Can you work these out from the model? Positions are in its coordinate system, mm. A direction names the side the tool comes from. Give positions to 0.01 mm unless a question says otherwise; leave off trailing zeros. Loops run counter-clockwise (first coordinate to the right, second up) from the corner with the lowest first, then second, coordinate; pieces in that order, holes last. Notation, with made-up numbers: (-9, -26) - (33, -26) arc R15 cw to (33, -6) - close; hole circle Ø7 at (19.25, 39.5). An arc over 180 degrees is marked (long way). Answer in a Markdown table with one row per item.
from build123d import *

# Parameters (mm, degrees)
BOSS_EXTRUDE1_DEPTH = 1500
CUT_EXTRUDE1_DEPTH  = 100
SKETCH3_R           = 50
CUT_EXTRUDE2_DEPTH  = 50
SKETCH4_R           = 25
CUT_EXTRUDE3_DEPTH  = 25


with BuildPart() as part:
    # Sketch1 → Boss-Extrude1 (new body)
    with BuildSketch(Plane(origin=(0, 0, 0), x_dir=(0, 0, -1), z_dir=(1, 0, 0))):
        with BuildLine():
            Line((-50, 50), (-50, -50))
            ThreePointArc((-50, -50), (0, -100), (50, -50))
            Line((50, -50), (50, 50))
            ThreePointArc((50, 50), (0, 100), (-50, 50))
        make_face()
    extrude(amount=-BOSS_EXTRUDE1_DEPTH)

    # Sketch2 → Cut-Extrude1 (cut)
    with BuildSketch(Plane.XY.offset(50)):
        with BuildLine():
            Line((-100.5, 100), (0, 100))
            Line((0, 100), (0, -100))
            Line((0, -100), (-100.5, -100))
            ThreePointArc((-100.5, -100), (-0.5, 0), (-100.5, 100))
        make_face()
    extrude(amount=-CUT_EXTRUDE1_DEPTH, mode=Mode.SUBTRACT)

    # Sketch3 → Cut-Extrude2 (cut)
    with BuildSketch(Plane.XY.offset(50)):
        with Locations((-100, 0)):
            Circle(SKETCH3_R)
    extrude(amount=-CUT_EXTRUDE2_DEPTH, mode=Mode.SUBTRACT)

    # Sketch4 → Cut-Extrude3 (cut)
    with BuildSketch(Plane.ZY.offset(1500)):
        with Locations((0, 50)):
            Circle(SKETCH4_R)
        with Locations((0, -50)):
            Circle(SKETCH4_R)
    extrude(amount=-CUT_EXTRUDE3_DEPTH, mode=Mode.SUBTRACT)


solid = part.part
Q1. For pin 1 (10 mm diameter, centred on x = -464.5, z = -15.5, fed in from +Y); pin 2 (3 mm diameter, centred on y = -28, z = 0.5, fed in from -X); pin 3 (1 mm diameter, centred on y = -2, z = 13.5, fed in from +X), each with a flat end and sliding along its axis, tell me the tip position at first contact or that it passes through.
Checked values:
| item | result |
|---|---|
| pin 1 | stops at y = 98.89 |
| pin 2 | stops at x = -1475 |
| pin 3 | stops at x = -0.51 |
Q2. Imagine slicing it at B-B, the plane x = -1196.5. Write out the boundary of the cut face in (y, z).
Checked values:
| item | result |
|---|---|
| outline | (-50, -50) - (50, -50) arc R50 ccw to (50, 50) - (-50, 50) arc R50 ccw to start |
Q3. If we mould it in two halves opening along Y, with no side actions, what happens to faces 4 (the face through (-790, 1, 50)), 5 (the face through (-1487.675, -74.406, -5.42)), 6 (the face through (-1487.675, 25.594, -5.42)), 7 (the face through (-0.524, -2.199, 0.7))? For each: released by +Y, released by -Y, zero draft, split by the parting line, or undercut.
Checked values:
| item | result |
|---|---|
| face 4 | zero draft |
| face 5 | undercut |
| face 6 | undercut |
| face 7 | split by the parting line |
Q4. If I drill on line 1 (Y direction, x = -1481.25, z = 0); line 2 (X direction, y = 2.5, z = 22); line 3 (X direction, y = 0, z = 37.5), over which ranges is the centre line in solid material (lowest first)? Write a range as [from, to].
Checked values:
| item | result |
|---|---|
| line 1 | y = [-100, -75], [-25, 25], [75, 100] |
| line 2 | x = [-1500, -149.94], [-50.06, -0.53] |
| line 3 | x = [-1500, -150], [-50, -0.5] |
Q5. Imagine slicing it at A-A, the plane y = 0. Write out the boundary of the cut face in (x, z).
Checked values:
| item | result |
|---|---|
| outline | (-1500, -50) - (-0.5, -50) - (-0.5, 50) - (-50, 50) - (-50, 0) - (-150, 0) - (-150, 50) - (-1500, 50) - close |
Q6. On a 3-axis mill with a long thin cutter (end or side, diameter ignored), from which of +Z, -Z, +X, -X, +Y, -Y can I reach the whole of each face in a straight line? I mean faces 1 (the face through (-740, -1, -50)), 2 (the face through (-1475, -50, 0)), 3 (the face through (-140, -30, 25)). Say none if no direction works.
Checked values:
| item | result |
|---|---|
| face 1 | -Z, +X, -X, +Y, -Y |
| face 2 | -X |
| face 3 | +Z |
